Read the model definition and answer for the solid it produces. Units are mm, in the model's axes. Face numbers are marked on the shaded views. A direction names the side the tool comes from. Round coordinates to 2 decimals unless told otherwise and drop trailing zeros. Order: outer loops, then holes, each group sorted by start corner. A loop starts at its lowest first (then second) coordinate and runs counter-clockwise, first axis right, second up. Notation, with made-up numbers: M 5.25,61 L 10.25,61 A19 cw 10.25,80 Z; hole C -28,68 d4. An arc over 180 degrees is marked long. Answer as CSV lines item,"result".
```python
from build123d import *

# Parameters (mm, degrees)
F0_W      = 152.4
F0_H      = 101.6
F1_DEPTH  = 25.4
F2_W      = 7.9375
F2_H      = 7.9375
F3_DEPTH  = 76.2
F4_W      = 7.9375
F4_H      = 7.9375
F7_DEPTH  = 76.2
F5_W      = 7.9375
F5_H      = 7.9375
F8_DEPTH  = 76.2
F6_W      = 7.9375
F6_H      = 7.9375
F9_DEPTH  = 76.2
F10_W     = 136.525
F10_H     = 85.725
F11_DEPTH = 12.7


# Not quite as in the source:
# - a length typed as a fraction of an inch, garbled in the dataset ("3 / 203.2 mm" for 3/8 in), is restored


with BuildPart() as f1:
    # F0 (on Front) → F1 (new body)
    with BuildSketch(Plane.XZ):
        with Locations((-82.3848899454, 39.5816343878)):
            Rectangle(F0_W, F0_H)
    extrude(amount=F1_DEPTH)

    # F2 (on face) → F3 (join)
    with BuildSketch(Plane.XZ.offset(25.4)):
        with Locations((-154.6161399454, 86.4128843878)):
            Rectangle(F2_W, F2_H)
    extrude(amount=F3_DEPTH)

    # F4 (on face) → F7 (join)
    with BuildSketch(Plane.XZ.offset(25.4)):
        with Locations((-10.1536399454, 86.4128843878)):
            Rectangle(F4_W, F4_H)
    extrude(amount=F7_DEPTH)

    # F5 (on face) → F8 (join)
    with BuildSketch(Plane.XZ.offset(25.4)):
        with Locations((-154.5934006572, -7.1469780084)):
            Rectangle(F5_W, F5_H)
    extrude(amount=F8_DEPTH)

    # F6 (on face) → F9 (join)
    with BuildSketch(Plane.XZ.offset(25.4)):
        with Locations((-11.0744582489, -6.1915257747)):
            Rectangle(F6_W, F6_H)
    extrude(amount=F9_DEPTH)

    # F10 (on face) → F11 (cut)
    with BuildSketch(Plane(origin=(0, 0, 0), x_dir=(-1, 0, 0), z_dir=(0, 1, 0))):
        with Locations((82.3848899454, 39.5816343878)):
            Rectangle(F10_W, F10_H)
    extrude(amount=-F11_DEPTH, mode=Mode.SUBTRACT)


solid = f1.part
```
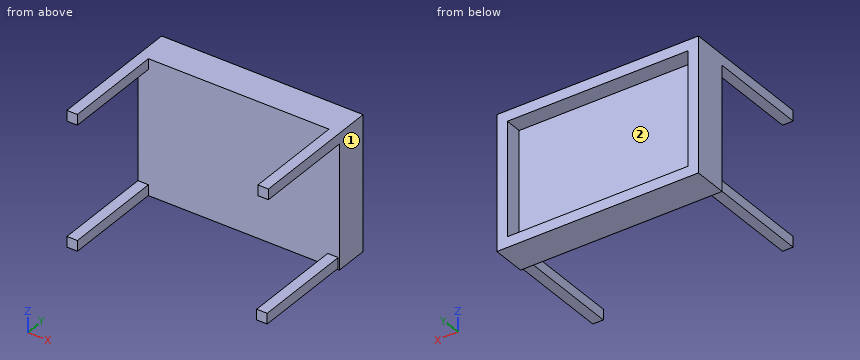
Item 1: A cutting plane is placed at C-C, the plane x = -71. Determine the outline of the cut face in (y, z), and give its area (3 significant figures).
Ans:
outline,"M -25.4,-11.22 L 0,-11.22 L 0,-3.28 L -12.7,-3.28 L -12.7,82.44 L 0,82.44 L 0,90.38 L -25.4,90.38 Z"
area,"1,490 mm2"
Item 2: A cutting plane is placed at A-A, the plane y = -49. Determine the outline of the cut face in (x, z).
Ans:
outline,"M -158.58,82.44 L -150.65,82.44 L -150.65,90.38 L -158.58,90.38 Z; M -158.56,-11.12 L -150.62,-11.12 L -150.62,-3.18 L -158.56,-3.18 Z; M -15.04,-10.16 L -7.11,-10.16 L -7.11,-2.22 L -15.04,-2.22 Z; M -14.12,82.44 L -6.18,82.44 L -6.18,90.38 L -14.12,90.38 Z"
Item 3: Find the intervals of material crossed by probe 1 along X at (y, z) = (-7.5, 19.5); probe 2 along Y at (x, z) = (-56.5, -6.5); probe 3 along Y at (x, z) = (-83, 64), in increasing order. Write a range as [from, to].
Ans:
probe 1,"[-158.58, -150.65], [-14.12, -6.18]"
probe 2,"[-25.4, 0]"
probe 3,"[-25.4, -12.7]"
Item 4: Flat-ended cylindrical pins translate along their axes: pin 1 (2.5 mm diameter, centred on x = -9.5, y = -54.5, fed in from -Z); pin 2 (2.5 mm diameter, centred on y = -74.5, z = -8, fed in from +X); pin 3 (2.5 mm diameter, centred on y = -77.5, z = -5.5, fed in from -X). Find the tip coordinate at first contact, or state that the pin passes through.
Ans:
pin 1,"z = -10.16"
pin 2,"x = -7.11"
pin 3,"x = -158.56"
Item 5: A cutting plane is placed at B-B, the plane z = 79.5. Determine the outline of the cut face in (x, y), and give its area (3 significant figures).
Ans:
outline,"M -158.58,-25.4 L -6.18,-25.4 L -6.18,0 L -14.12,0 L -14.12,-12.7 L -150.65,-12.7 L -150.65,0 L -158.58,0 Z"
area,"2,140 mm2"
Item 6: A tool of negligible diameter and unlimited length cuts with its end or side. For the marked faces 1 and 2, from which of +Z, -Z, +X, -X, +Y, -Y can it reach the whole face along a straight path? Write none if from no direction.
Ans:
face 1,"+Z, -Z, +X, +Y, -Y"
face 2,"+Y"
